Autodesk Inventor part; units mm, degrees
ref_plane "YZ Plane" through (0, 0, 0) normal (1, 0, 0) x (0, 1, 0)
ref_plane "XZ Plane" through (0, 0, 0) normal (0, 1, 0) x (-1, 0, 0)
ref_plane "XY Plane" through (0, 0, 0) normal (0, 0, 1) x (1, 0, 0)
sketch "Sketch2" plane through (0, 0, 0) normal (0, 0, 1) x (1, 0, 0)
  line L0 (0, -40) -> (0, -15)
  line L1 (0, -15) -> (-34, -15)
  line L2 (-34, -15) -> (-34, 58)
  line L3 (-34, 58) -> (34, 58)
  line L4 (34, 58) -> (34, -15)
  line L5 (34, -15) -> (0, -15)
  circle A0 centre (-34, 58) radius 1.5
  circle A1 centre (34, 58) radius 1.5
  circle A2 centre (-34, -15) radius 1.5
  circle A3 centre (34, -15) radius 1.5
  line L6 (32.5, 56.5) -> (-32.5, 56.5)
  line L7 (-32.5, 56.5) -> (-32.5, -13.5)
  line L8 (-32.5, -13.5) -> (0, -13.5)
  line L9 (0, -13.5) -> (32.5, -13.5)
  line L10 (32.5, -13.5) -> (32.5, 56.5)
  line L11 (37, -18) -> (37, 61)
  line L12 (37, 61) -> (-37, 61)
  line L13 (-37, 61) -> (-37, -18)
  line L14 (-37, -18) -> (0, -18)
  line L15 (0, -18) -> (37, -18)
  point P0 (0, 0)
  dimension "d0" = 25
  dimension "d1" = 34
  dimension "d3" = 68
  dimension "d4" = 3
  dimension "d5" = 3
  dimension "d6" = 3
  dimension "d11" = 1.5
  dimension "d13" = 3
extrude "Extrusion1" add sketch "Sketch2" along normal blind 20 contours L1 A2 L2 A0 L3 A1 L4 A3 L5 | L15 L14 L13 L12 L11
fillet "Fillet1" radius 2 4 edges at (37, -18, 10) (37, 61, 10) (-37, 61, 10) (-37, -18, 10)
sketch "Sketch3" plane through (0, 0, 20) normal (0, 0, 1) x (1, 0, 0)
  arc A0 (-37, -16) -> (-35, -18) centre (-35, -16) ccw
  line L0 (-35, -18) -> (35, -18)
  arc A1 (35, -18) -> (37, -16) centre (35, -16) ccw
  line L1 (37, -16) -> (37, 59)
  arc A2 (37, 59) -> (35, 61) centre (35, 59) ccw
  line L2 (35, 61) -> (-35, 61)
  arc A3 (-35, 61) -> (-37, 59) centre (-35, 59) ccw
  line L3 (-37, 59) -> (-37, -16)
  circle A4 centre (34, -15) radius 1.5
  circle A5 centre (-34, -15) radius 1.5
  circle A6 centre (-34, 58) radius 1.5
  line L4 (32.5, 56.5) -> (32.5, -13.5)
  line L5 (32.5, -13.5) -> (-32.5, -13.5)
  line L6 (-32.5, -13.5) -> (-32.5, 56.5)
  line L7 (-32.5, 56.5) -> (32.5, 56.5)
  circle A7 centre (34, 58) radius 1.5
  point P0 (0, 0)
extrude "Extrusion2" add sketch "Sketch3" along normal blind 3 contours L3 A3 L2 A2 L1 A1 L0 A0 | L4 L5 L6 L7
fillet "Fillet2" radius 1.5 8 edges at (36.4142, 60.4142, 23) (0, 61, 23) (-36.4142, 60.4142, 23) (-37, 21.5, 23) (-36.4142, -17.4142, 23) (0, -18, 23) (36.4142, -17.4142, 23) (37, 21.5, 23)
sketch "Sketch4" plane through (0, 0, 20) normal (0, 0, -1) x (-1, 0, 0)
  line L0 (-32.5, 56.5) -> (-32.5, -13.5)
  line L1 (-32.5, 56.5) -> (-12.5, 56.5)
  line L2 (32.5, 56.5) -> (-32.5, 56.5)
  line L3 (-12.5, 56.5) -> (-12.5, 42.5)
  line L4 (-12.5, 42.5) -> (-32.5, 42.5)
  point P0 (0, 0)
  dimension "d18" = 20
  dimension "d19" = 14
extrude "Extrusion3" cut sketch "Sketch4" against normal blind 3
fillet "Fillet3" radius 1.5 4 edges at (12.5, 49.5, 23) (22.5, 56.5, 23) (32.5, 49.5, 23) (22.5, 42.5, 23)
sketch "Sketch6" plane through (0, 0, 23) normal (0, 0, 1) x (1, 0, 0)
  line L0 (34, -16.5) -> (-34, -16.5)
  line L1 (-35.5, -15) -> (-35.5, 58)
  line L2 (0, 21.5) -> (0, 36.5)
  line L3 (0, 36.5) -> (-15, 36.5)
  line L4 (-15, 36.5) -> (-15, 6.5)
  line L5 (-15, 6.5) -> (15, 6.5)
  line L6 (15, 6.5) -> (15, 36.5)
  line L7 (15, 36.5) -> (0, 36.5)
  line L8 (-12, 33.5) -> (0, 33.5)
  line L9 (0, 33.5) -> (12, 33.5)
  line L10 (12, 33.5) -> (12, 9.5)
  line L11 (12, 9.5) -> (-12, 9.5)
  line L12 (-12, 9.5) -> (-12, 33.5)
  line L13 (-15, 36.5) -> (-22.5, 36.5)
  circle A0 centre (-22.5, 36.5) radius 1.5
  circle A1 centre (-22.5, 6.5) radius 1.5
  circle A2 centre (22.5, 36.5) radius 1.5
  circle A3 centre (22.5, 6.5) radius 1.5
  dimension "d33" = 15
  dimension "d34" = 15
  dimension "d35" = 30
  dimension "d36" = 30
  dimension "d37" = 3
  dimension "d38" = 7.5
  dimension "d39" = 3
  dimension "d40" = 3
extrude "Extrusion5" cut sketch "Sketch6" against normal blind 5 contours L8 L9 L10 L11 L12 | A0 | A1 | A2 | A3
sketch "Sketch7" plane through (0, 0, 0) normal (0, 0, -1) x (-1, 0, 0)
  line L0 (32.5, -13.5) -> (32.5, 56.5)
  line L1 (32.5, 56.5) -> (27.5, 56.5)
  line L2 (32.5, 56.5) -> (-32.5, 56.5)
  line L3 (27.5, 56.5) -> (29.5, 56.5)
  line L4 (29.5, 56.5) -> (29.5, 58.5)
  line L5 (29.5, 58.5) -> (25.5, 58.5)
  line L6 (25.5, 58.5) -> (25.5, 56.5)
  line L7 (29.5, 58.5) -> (31, 58.5)
  line L8 (31, 58.5) -> (31, 56.5)
  line L9 (25.5, 58.5) -> (24, 58.5)
  line L10 (24, 58.5) -> (24, 56.5)
  line L11 (0, 56.5) -> (0, 48.9008)
  line L12 (-32.5, 56.5) -> (-27.5, 56.5)
  line L13 (-32.5, 56.5) -> (32.5, 56.5)
  line L14 (-27.5, 56.5) -> (-29.5, 56.5)
  line L15 (-29.5, 56.5) -> (-29.5, 58.5)
  line L16 (-29.5, 58.5) -> (-25.5, 58.5)
  line L17 (-25.5, 58.5) -> (-25.5, 56.5)
  line L18 (-29.5, 58.5) -> (-31, 58.5)
  line L19 (-31, 58.5) -> (-31, 56.5)
  line L20 (-25.5, 58.5) -> (-24, 58.5)
  line L21 (-24, 58.5) -> (-24, 56.5)
  line L22 (24, 58.5) -> (-24, 58.5)
  point P0 (0, 0)
  dimension "d44" = 5
  dimension "d45" = 2
  dimension "d46" = 2
  dimension "d47" = 4
  dimension "d48" = 1.5
  dimension "d49" = 1.5
extrude "Extrusion6" cut sketch "Sketch7" against normal up to surface (20 mm away)
fillet "Fillet5" radius 1.5 4 edges at (31, 58.5, 10) (31, 56.5, 10) (-31, 58.5, 10) (-31, 56.5, 10)
sketch "Sketch8" plane through (37, -16, 0) normal (1, 0, 0) x (0, 0, -1)
  line L0 (0, 77) -> (-21.5, 77)
  line L1 (-10.75, 77) -> (-10.75, -2)
  line L2 (-21.5, -2) -> (0, -2)
  circle A0 centre (-10.75, 37.5) radius 2
  point P0 (0, 16)
  dimension "d54" = 4
extrude "Extrusion7" cut sketch "Sketch8" against normal through all
properties part number "manta ray battery pack"
Geometry check sheet. Reference: the model listing, model coordinates, mm. A direction names the side the tool comes from. Round coordinates to 2 decimals unless told otherwise and drop trailing zeros. Order: outer loops, then holes, each group sorted by start corner. A loop starts at its lowest first (then second) coordinate and runs counter-clockwise, first axis right, second up. Notation, with made-up numbers: M 65,-25.5 L 90,-25.5 A12 cw 90,-5.5 Z; hole C 18,24.5 d3. An arc over 180 degrees is marked long. Write each question's results on one line, items separated by ' | '. Start each with the question number.
1. Cross-section at A-A on y = 36.5. Record the boundary of the cut face in (x, z).
2. Draft check along Y on faces 1 (the face through (37, 21, 8)), 2 (the face through (-36.4, 60.43, 10.9)), 3 (the face through (23, 56.5, 21)). Enter one of: pulls with the +Y half, pulls with the -Y half, needs draft (parallel to the pull), parting line crosses it, or undercut.
3. Material ranges on L1, parallel to Y at x = 24, z = 1.75; L2, parallel to Y at x = -34, z = 8.5; L3, parallel to X at y = 39, z = 10, recorded low to high. Write a range as from..to.
4. Cross-section at C-C on z = 1.5. Record the boundary of the cut face in (x, y).
5. Cross-section at D-D on x = -34. Give the number of separate pieces and of enclosed holes in the cut face, plus the area to 3 significant figures.
6. Set-up check for faces 4 (the face through (-15, 23, 20)), 5 (the face through (-34.719, 22.852, 12.224)), 6 (the face through (0, 9.5, 22)): record each of +Z, -Z, +X, -X, +Y, -Y from which the full face is reachable in a straight line by a thin tool's end or side.
7. Go/stop test with a flat-tipped pin: P1, Ø4, axis at x = 8, y = -1, coming from the -Z side. Record where the tip stops, or that it passes through.
8. Cross-section at B-B on x = 22.5. Record the boundary of the cut face in (y, z), plus the area to 3 significant figures.
Resolved:
1) outline: M -37,0 L -32.5,0 L -32.5,20 L -24,20 L -24,23 L -35.5,23 A1.5 ccw -37,21.5 Z; M -21,20 L 21,20 L 21,23 L -21,23 Z; M 24,20 L 32.5,20 L 32.5,0 L 37,0 L 37,21.5 A1.5 ccw 35.5,23 L 24,23 Z
2) face 1: needs draft | face 2: pulls with the +Y half | face 3: undercut
3) L1: -18..-13.5, 58.5..61 | L2: -18..-16.5, -13.5..56.5, 59.5..61 | L3: -37..-32.5, 32.5..37
4) outline: M -37,-16 A2 ccw -35,-18 L 35,-18 A2 ccw 37,-16 L 37,59 A2 ccw 35,61 L -35,61 A2 ccw -37,59 Z; hole C -34,-15 d3; hole C -34,58 d3; hole M -32.5,-13.5 L 32.5,-13.5 L 32.5,56.5 L 32.33,56.5 A1.5 cw 30.91,57.5 A1.5 ccw 29.5,58.5 L -29.5,58.5 A1.5 ccw -30.91,57.5 A1.5 cw -32.33,56.5 L -32.5,56.5 Z; hole C 34,-15 d3; hole C 34,58 d3
5) separate pieces: 3 | enclosed holes: 1 | area: 1,670 mm2
6) face 4: -Z | face 5: +X, -X | face 6: +Z, -Z
7) P1: z = 20
8) outline: M -18,0 L -13.5,0 L -13.5,20 L 5,20 L 5,23 L -16.5,23 A1.5 ccw -18,21.5 Z; M 8,20 L 35,20 L 35,23 L 8,23 Z; M 38,20 L 42.5,20 L 42.5,21.5 A1.5 ccw 41,23 L 38,23 Z; M 56.5,20 L 58.5,20 L 58.5,0 L 61,0 L 61,21.5 A1.5 ccw 59.5,23 L 58,23 A1.5 ccw 56.5,21.5 Z | area: 315 mm2
